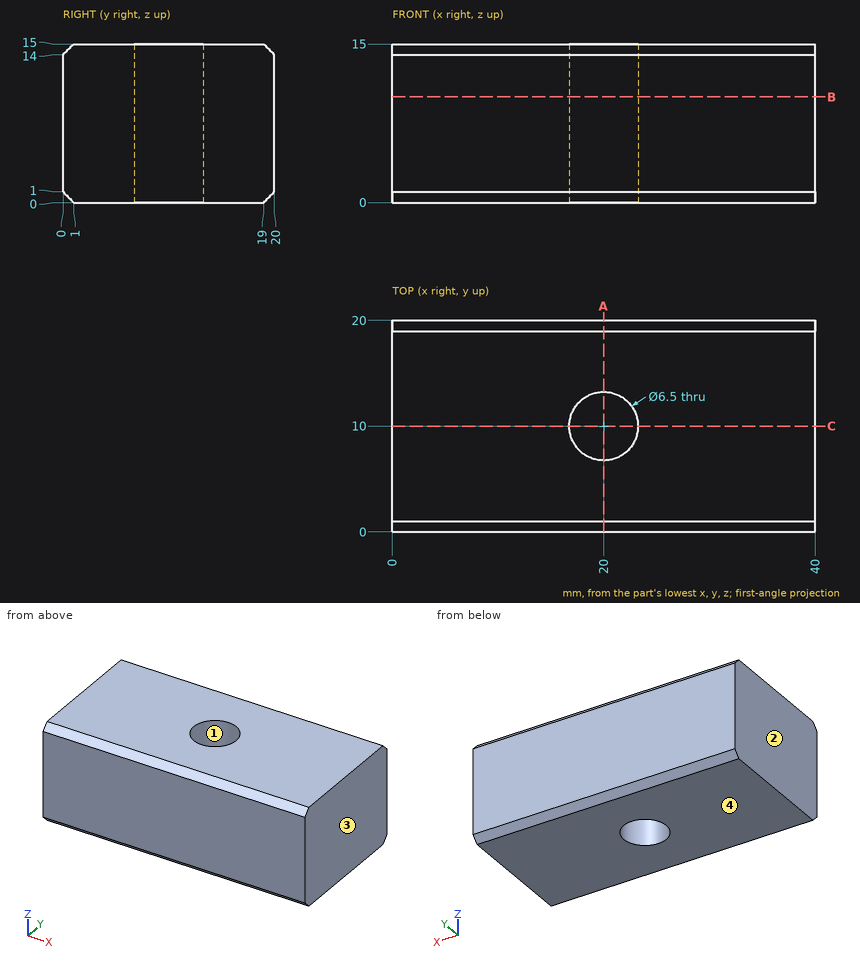
Geometry: see drawing. Coordinates: mm, zero at the bounding-box minimum. Give positions to 0.01 mm unless a question says otherwise; leave off trailing zeros. Write each loop counter-clockwise with the first axis right and the second up, starting at its lowest first coordinate (ties: lowest second). Pieces come first, ordered by that corner, then holes. Notation, with made-up numbers: M 67.25,11.25 L 84.25,11.25 A14 ccw 84.25,30.25 Z; hole C 27,-21.75 d6. An arc over 180 degrees is marked long. Return JSON: item names as keys, results as strings. Group by question number.
1) Cut plane B-B, the plane z = 10. Output: boundary loops of the cut face in (x, y).
2) Cut plane A-A, the plane x = 20. Output: boundary loops of the cut face in (y, z).
3) Cut plane C-C, the plane y = 10. Output: boundary loops of the cut face in (x, z).
4) Ray query, L1, parallel to Y at x = 20, z = 3.25; L2, parallel to X at y = 7, z = 10.5; L3, parallel to Y at x = 22, z = 6.5. Return the intervals inside material, ascending.
5) Draft query along X for the marked faces 1, 2, 3 and 4. Return one class per face: released by +X, released by -X, zero draft, split by the parting line, or undercut.
Data:
{
 "1": {"outline": "M 0,0 L 40,0 L 40,20 L 0,20 Z; hole C 20,10 d6.5"},
 "2": {"outline": "M 0,1 L 1,0 L 6.75,0 L 6.75,15 L 1,15 L 0,14 Z; M 13.25,0 L 19,0 L 20,1 L 20,14 L 19,15 L 13.25,15 Z"},
 "3": {"outline": "M 0,0 L 16.75,0 L 16.75,15 L 0,15 Z; M 23.25,0 L 40,0 L 40,15 L 23.25,15 Z"},
 "4": {"L1": "y = 0 to 6.75, 13.25 to 20", "L2": "x = 0 to 18.75, 21.25 to 40", "L3": "y = 0 to 7.44, 12.56 to 20"},
 "5": {"face 1": "undercut", "face 2": "released by -X", "face 3": "released by +X", "face 4": "zero draft"}
}
